Design review of the part built by this model. Coordinates are the model's own, in mm. A direction names the side the tool comes from. Give positions to 0.01 mm unless a question says otherwise; leave off trailing zeros. Loops run counter-clockwise (first coordinate to the right, second up) from the corner with the lowest first, then second, coordinate; pieces in that order, holes last. Notation, with made-up numbers: (78.5, 49.5) -> (103.5, 49.5) arc R22 cw to (103.5, 61.5) -> close; hole circle Ø3 at (21, 89). An arc over 180 degrees is marked (long way). Answer as CSV lines item,"result".
from build123d import *

# Parameters (mm, degrees)
F0_W     = 20
F0_H     = 16
F1_DEPTH = 11.5
F2_W     = 12
F2_H     = 50
F3_DEPTH = 6
F4_R     = 0.5


with BuildPart() as f1:
    # F0 (on Top) → F1 (new body)
    with BuildSketch(Plane.XY):
        Rectangle(F0_W, F0_H)
    extrude(amount=F1_DEPTH)

    # F2 (on Top) → F3 (join)
    with BuildSketch(Plane.XY):
        with Locations((0, -33)):
            Rectangle(F2_W, F2_H)
    extrude(amount=F3_DEPTH)

    # F4
    f4_edges = [f1.edges().sort_by_distance(p)[0] for p in [
        (10, 0, 0),
        (0, 8, 0),
        (-10, 0, 0),
        (-8, -8, 0),
        (-6, -33, 0),
        (0, -58, 0),
        (6, -33, 0),
        (8, -8, 0),
        (10, 0, 11.5),
        (0, 8, 11.5),
        (-10, 0, 11.5),
        (0, -8, 11.5),
        (6, -33, 6),
        (0, -8, 6),
        (-6, -33, 6),
        (0, -58, 6),
        (10, 8, 5.75),
        (-10, 8, 5.75),
        (-6, -8, 3),
        (6, -8, 3),
        (10, -8, 5.75),
        (-10, -8, 5.75),
    ]]
    fillet(f4_edges, radius=F4_R)


solid = f1.part
Q1. For faces 1 (the flat face through (6, -34, 3)), 2 (the flat face through (-6, -34, 3)), 3 (the flat face through (0, -33, 6)), list the 3-axis set-ups (+Z, -Z, +X, -X, +Y, -Y) from which the entire face can be reached by the end or side of a thin tool; tool diameter is ignored.
Filled sheet:
face 1,"+Z, -Z, +X, -Y"
face 2,"+Z, -Z, -X, -Y"
face 3,"+Z, +X, -X, -Y"
Q2. To check wall thickness, follow probe 1 along Y at (x, z) = (-8, 8.25); probe 2 along X at (y, z) = (-40, 4); probe 3 along Z at (x, y) = (3.75, -25). State the ranges of each line that lie inside material, in increasing order. Write a range as from..to.
Filled sheet:
probe 1,"y = -8..8"
probe 2,"x = -6..6"
probe 3,"z = 0..6"
Q3. We need section B-B, the plane z = 4.75. State the section outline as (x, y) points, and give its area (3 significant figures).
Filled sheet:
outline,"(-10, -7.5) arc R0.5 ccw to (-9.5, -8) -> (-6.5, -8) arc R0.5 cw to (-6, -8.5) -> (-6, -58) -> (6, -58) -> (6, -8.5) arc R0.5 cw to (6.5, -8) -> (9.5, -8) arc R0.5 ccw to (10, -7.5) -> (10, 7.5) arc R0.5 ccw to (9.5, 8) -> (-9.5, 8) arc R0.5 ccw to (-10, 7.5) -> close"
area,"920 mm^2"
Q4. We need section D-D, the plane x = -1.75. State the section outline as (y, z) points.
Filled sheet:
outline,"(-58, 0.5) arc R0.5 ccw to (-57.5, 0) -> (7.5, 0) arc R0.5 ccw to (8, 0.5) -> (8, 11) arc R0.5 ccw to (7.5, 11.5) -> (-7.5, 11.5) arc R0.5 ccw to (-8, 11) -> (-8, 6.5) arc R0.5 cw to (-8.5, 6) -> (-57.5, 6) arc R0.5 ccw to (-58, 5.5) -> close"
Q5. We need section C-C, the plane y = -43. State the section outline as (x, z) points, and give its area (3 significant figures).
Filled sheet:
outline,"(-6, 0.5) arc R0.5 ccw to (-5.5, 0) -> (5.5, 0) arc R0.5 ccw to (6, 0.5) -> (6, 5.5) arc R0.5 ccw to (5.5, 6) -> (-5.5, 6) arc R0.5 ccw to (-6, 5.5) -> close"
area,"71.8 mm^2"
Q6. We need section A-A, the plane x = 7.5. State the section outline as (y, z) points.
Filled sheet:
outline,"(-8, 0.5) arc R0.5 ccw to (-7.5, 0) -> (7.5, 0) arc R0.5 ccw to (8, 0.5) -> (8, 11) arc R0.5 ccw to (7.5, 11.5) -> (-7.5, 11.5) arc R0.5 ccw to (-8, 11) -> close"
Q7. Clearance check with flat-ended pins moving along their axes: pin 1 Ø1.5 at (y, z) = (-40, 4) entering from -X; pin 2 Ø1.5 at (y, z) = (-43, 7.5) entering from +X; pin 3 Ø3.5 at (x, y) = (0, -44.5) entering from +Z; pin 4 Ø2.5 at (y, z) = (-29.5, 3.5) entering from +X. State where each tip first meets the part, or that it passes through.
Filled sheet:
pin 1,"stops at x = -6"
pin 2,"passes through"
pin 3,"stops at z = 6"
pin 4,"stops at x = 6"
